Drawing for the job (mm, zero at the part's lowest x, y, z). A direction names the side the tool comes from. Give positions to 0.01 mm unless a question says otherwise; leave off trailing zeros. Order: outer loops, then holes, each group sorted by start corner. A loop starts at its lowest first (then second) coordinate and runs counter-clockwise, first axis right, second up. Notation, with made-up numbers: (62, 57) - (113, 57) arc R23 ccw to (113, 89) - close; hole circle Ø9 at (-5.75, 65). An arc over 180 degrees is marked (long way). Use a Markdown table: item, result. Add a question column.
(1) Slice it at D-D (x = 20). Write the cut outline in (y, z), then the cut area to 3 significant figures.
(2) Wall check: line 1 (Y direction, x = 2.75, z = 3.6); line 2 (Z direction, x = 4, y = 2.45); line 3 (X direction, y = 2.6, z = 4.5). Give the ranges that are in metal, low to high.
(3) Which spindle directions (+Z, -Z, +X, -X, +Y, -Y) get a long thin tool onto all of the face, cutting with end or side? Do the marked faces 1 and 2. Say none if no direction does.
(4) Slice it at C-C (z = 3.2). Write the cut outline in (x, y), then the cut area to 3 significant figures.
(5) Slice it at A-A (y = 2). Write the cut outline in (x, z).
(6) Flat gauge pins, fed straight in: pin 1 (2 mm diameter, centred on x = 12, y = 2.5, fed in from -Z); pin 2 (1.4 mm diameter, centred on x = 2.75, y = 2, fed in from +Z). Where does each tip first touch, or does it go through?
(7) Mould opens along X. For the marked faces 3, 4 and 5 say: +X half, -X half, draft (parallel to the pull), parting line (faces both ways), or undercut.
(8) Slice it at B-B (x = 2.75). Write the cut outline in (y, z), then the cut area to 3 significant figures.
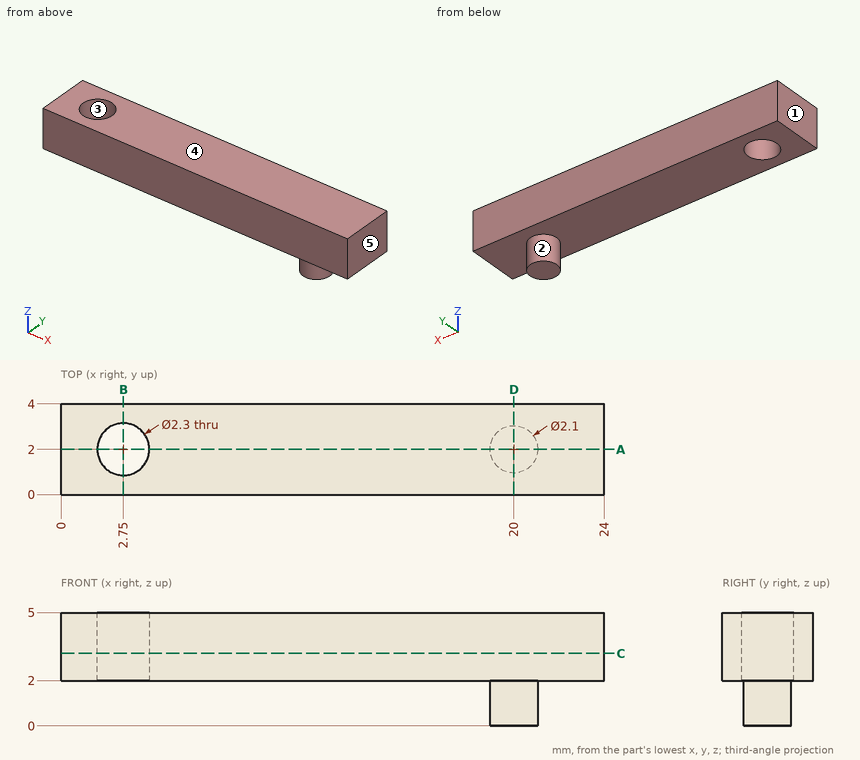
Solution:
| question | item | result |
|---|---|---|
| 1 | outline | (0, 2) - (0.95, 2) - (0.95, 0) - (3.05, 0) - (3.05, 2) - (4, 2) - (4, 5) - (0, 5) - close |
| 1 | area | 16.2 mm2 |
| 2 | line 1 | 0 to 0.85, 3.15 to 4 |
| 2 | line 2 | 2 to 5 |
| 2 | line 3 | 0 to 1.77, 3.73 to 24 |
| 3 | face 1 | +Z, -Z, -X, +Y, -Y |
| 3 | face 2 | -Z |
| 4 | outline | (0, 0) - (24, 0) - (24, 4) - (0, 4) - close; hole circle Ø2.3 at (2.75, 2) |
| 4 | area | 91.8 mm2 |
| 5 | outline | (0, 2) - (1.6, 2) - (1.6, 5) - (0, 5) - close; (3.9, 2) - (18.95, 2) - (18.95, 0) - (21.05, 0) - (21.05, 2) - (24, 2) - (24, 5) - (3.9, 5) - close |
| 6 | pin 1 | z = 2 |
| 6 | pin 2 | through |
| 7 | face 3 | undercut |
| 7 | face 4 | draft |
| 7 | face 5 | +X half |
| 8 | outline | (0, 2) - (0.85, 2) - (0.85, 5) - (0, 5) - close; (3.15, 2) - (4, 2) - (4, 5) - (3.15, 5) - close |
| 8 | area | 5.10 mm2 |
